Input: part model. Units: mm. Frame: model coordinates. A direction names the side the tool comes from. Coordinates: 2 decimals unless noted, no trailing zeros. Order: outer loops, then holes, each group sorted by start corner. A loop starts at its lowest first (then second) coordinate and runs counter-clockwise, first axis right, second up. Notation, with made-up numbers: (15.5, 12) -> (47.5, 12) arc R25 cw to (47.5, 37) -> close; hole circle Ø5 at (-25.5, 43). An arc over 180 degrees is marked (long way). One line per question, with ' | ' between items.
```python
from build123d import *

# Parameters (mm, degrees)
BOSS_EXTRUDE1_DEPTH = 100
SKETCH2_R           = 5
CUT_EXTRUDE1_DEPTH  = 61
BOSS_EXTRUDE3_DEPTH = 70
BOSS_EXTRUDE4_REACH = 124.997
SKETCH4_W           = 48
SKETCH4_H           = 70
CUT_EXTRUDE2_REACH  = 131.834
FILLET1_R           = 10
CUT_EXTRUDE3_DEPTH  = 56
FILLET3_R           = 18
FILLET4_R           = 15
FILLET5_R           = 15


with BuildPart() as part:
    # Sketch1 → Boss-Extrude1 (new body)
    with BuildSketch(Plane(origin=(0, 0, 0), x_dir=(0, 0, -1), z_dir=(1, 0, 0))):
        Polygon((9.31960102, -5.422823355), (-6.40194197, 19.363300607), (-0.164443236, 19.363300607), (44.235722397, -50.636699393), (37.998223663, -50.636699393), (29.951005386, -37.94969088), align=None)
    extrude(amount=BOSS_EXTRUDE1_DEPTH)

    # Sketch2 → Cut-Extrude1 (cut)
    with BuildSketch(Plane(origin=(0, 0, -44.235722397), x_dir=(-1, 0, 0), z_dir=(0, 0, -1))):
        with Locations(Location((-80, -41.23638567, 0), (0, 0, 270))):
            Circle(SKETCH2_R)
        with Locations(Location((-20, -41.23638567, 0), (0, 0, 270))):
            Circle(SKETCH2_R)
        with Locations(Location((-20, 8.76361433, 0), (0, 0, 270))):
            Circle(SKETCH2_R)
        with Locations(Location((-80, 8.76361433, 0), (0, 0, 270))):
            Circle(SKETCH2_R)
    extrude(amount=-CUT_EXTRUDE1_DEPTH, mode=Mode.SUBTRACT)

    # Boss-Extrude4: up to this face of the body (flat: up to its plane)
    boss_extrude4_end = Plane(part.part.faces().sort_by_distance((50, -15.608520887, -15.780267556))[0])
    # Sketch4 → Boss-Extrude4 (add, up to the picked face)
    with BuildSketch(Plane(origin=(0, 0, 6.40194197), x_dir=(-1, 0, 0), z_dir=(0, 0, -1)), mode=Mode.PRIVATE) as boss_extrude4_sk1:
        with Locations((-50, -15.636699393)):
            Rectangle(SKETCH4_W, SKETCH4_H)
    boss_extrude4_tool1 = split(extrude(boss_extrude4_sk1.sketch, amount=BOSS_EXTRUDE4_REACH, mode=Mode.PRIVATE), bisect_by=boss_extrude4_end, keep=Keep.BOTH, mode=Mode.PRIVATE)


with BuildPart() as body_2:
    # Sketch3 → Boss-Extrude3 (new body)
    with BuildSketch(Plane(origin=(0, 19.363300607, 0), x_dir=(1, 0, 0), z_dir=(0, 1, 0))):
        with BuildLine():
            Line((26, -6.40194197), (74, -6.40194197))
            ThreePointArc((74, -6.40194197), (50, -10.164443236), (26, -6.40194197))
        make_face()
    extrude(amount=-BOSS_EXTRUDE3_DEPTH)


with BuildPart() as part_1:
    add(part.part)

    add(body_2.part)  # Boss-Extrude4 merges body 2
    add(boss_extrude4_tool1.solids().sort_by(Axis((50, -15.636699, 6.401942), (0, 0, -1)))[0])

    # Cut-Extrude2: up to this face of the body (flat: up to its plane)
    cut_extrude2_end = Plane(part_1.part.faces().sort_by_distance((87.661220736, -15.580052964, -15.762210692))[0])
    # Sketch5 → Cut-Extrude2 (cut, up to the picked face)
    with BuildSketch(Plane.XZ.offset(50.636699393), mode=Mode.PRIVATE) as cut_extrude2_sk1:
        with BuildLine():
            Line((68.503998914, -37.998223663), (31.496001086, -37.998223663))
            Line((31.496001086, -37.998223663), (31.496001086, 4.779601344))
            ThreePointArc((31.496001086, 4.779601344), (50, 7.087022557), (68.503998914, 4.779601344))
            Line((68.503998914, 4.779601344), (68.503998914, -37.998223663))
        make_face()
    cut_extrude2_tool1 = split(extrude(cut_extrude2_sk1.sketch, amount=-CUT_EXTRUDE2_REACH, mode=Mode.PRIVATE), bisect_by=cut_extrude2_end, keep=Keep.BOTH, mode=Mode.PRIVATE)
    add(cut_extrude2_tool1.solids().sort_by(Axis((50, -50.636699, -15.832469), (0, 1, 0)))[0], mode=Mode.SUBTRACT)

    # Fillet1
    # the kernel refuses this fillet: 10 mm, written as the material it takes off along each edge
    with BuildSketch(Plane(origin=(100, -50.636699393, -69.235722397), x_dir=(-1, 0, 0), z_dir=(0, 0, 1)), Plane(origin=(100, 19.363300607, 31.40194197), x_dir=(-1, 0, 0), z_dir=(0, 0, -1))) as fillet1_piece_1:
        with BuildLine():
            CenterArc((FILLET1_R, -FILLET1_R), FILLET1_R, 90, 90)
            Line((0, -FILLET1_R), (0, 0))
            Line((0, 0), (FILLET1_R, 0))
        make_face()
    extrude(amount=56.237498734, mode=Mode.SUBTRACT)
    with BuildSketch(Plane(origin=(0, -50.636699393, -69.235722397), x_dir=(1, 0, 0), z_dir=(0, 0, 1)), Plane(origin=(0, 19.363300607, 31.40194197), x_dir=(1, 0, 0), z_dir=(0, 0, -1))) as fillet1_piece_2:
        with BuildLine():
            CenterArc((FILLET1_R, FILLET1_R), FILLET1_R, 180, 90)
            Line((0, FILLET1_R), (0, 0))
            Line((0, 0), (FILLET1_R, 0))
        make_face()
    extrude(amount=56.237498734, mode=Mode.SUBTRACT)

    # Sketch7 → Cut-Extrude3 (cut)
    with BuildSketch(Plane(origin=(74, 0, 0), x_dir=(0, 0, -1), z_dir=(1, 0, 0))):
        Polygon((5.879968804, 0), (-34.029101203, 0), (-34.029101203, -30), (24.908611218, -30), align=None)
    extrude(amount=-CUT_EXTRUDE3_DEPTH, mode=Mode.SUBTRACT)

    # Fillet3
    # the kernel refuses this fillet: 18 mm, written as the material it takes off along each edge
    with BuildSketch(Plane(origin=(74, 60.763896609, 6.40194197), x_dir=(-0.9790132085588953, 0, 0.20379680435967867), z_dir=(0, -1, 0))) as fillet3_piece_1_section:
        with BuildLine():
            CenterArc((14.659822692, 17.8993972), FILLET3_R, 191.759074187, 84.301431918)
            Line((-2.962415062, 14.231054722), (0, 0))
            ThreePointArc((0, 0), (8.2801192, -0.43832682), (16.560238401, 0))
        make_face()
    fillet3_piece_1 = extrude(amount=102.16449261, mode=Mode.PRIVATE)
    fillet3_piece_1 = split(fillet3_piece_1, bisect_by=Plane(origin=(69.993439145, 10.97404697, 1.080738384), z_dir=(0, -0.5356273864218708, 0.8444544409942292)), keep=Keep.TOP, mode=Mode.PRIVATE)
    add(fillet3_piece_1, mode=Mode.SUBTRACT)
    with BuildSketch(Plane(origin=(74, 11.400596002, 6.40194197), x_dir=(-0.9790132085588953, 0, 0.2037968043596786), z_dir=(0, -1, 0))) as fillet3_piece_2_section:
        with BuildLine():
            CenterArc((14.659822692, 17.8993972), FILLET3_R, 191.759074187, 84.301431918)
            Line((-2.962415062, 14.231054722), (0, 0))
            ThreePointArc((0, 0), (8.2801192, -0.43832682), (16.560238401, 0))
        make_face()
    fillet3_piece_2 = extrude(amount=103.437891396, mode=Mode.PRIVATE)
    fillet3_piece_2 = split(fillet3_piece_2, bisect_by=Plane(origin=(70.341248141, 8.727743457, -0.34406516), z_dir=(0, -0.5356273864218708, 0.8444544409942292)), keep=Keep.TOP, mode=Mode.PRIVATE)
    add(fillet3_piece_2, mode=Mode.SUBTRACT)
    with BuildSketch(Plane(origin=(26, 11.400596002, 6.40194197), x_dir=(0, 0, -1), z_dir=(0, -1, 0))) as fillet3_piece_3_section:
        with BuildLine():
            CenterArc((14.536121267, 18), FILLET3_R, 185.698568082, 84.301431918)
            ThreePointArc((-3.374923665, 16.212692131), (-2.116589579, 8.01701646), (0, 0))
            Line((0, 0), (14.536121267, 0))
        make_face()
    fillet3_piece_3 = extrude(amount=103.437891396, mode=Mode.PRIVATE)
    fillet3_piece_3 = split(fillet3_piece_3, bisect_by=Plane(origin=(29.658751859, 8.727743457, -0.344065159), z_dir=(0, -0.5356273864218708, 0.8444544409942292)), keep=Keep.TOP, mode=Mode.PRIVATE)
    add(fillet3_piece_3, mode=Mode.SUBTRACT)
    with BuildSketch(Plane(origin=(26, 60.763896609, 6.40194197), x_dir=(0, 0, -1), z_dir=(0, -1, 0))) as fillet3_piece_4_section:
        with BuildLine():
            CenterArc((14.536121267, 18), FILLET3_R, 185.698568082, 84.301431918)
            ThreePointArc((-3.374923665, 16.212692131), (-2.116589579, 8.01701646), (0, 0))
            Line((0, 0), (14.536121267, 0))
        make_face()
    fillet3_piece_4 = extrude(amount=102.16449261, mode=Mode.PRIVATE)
    fillet3_piece_4 = split(fillet3_piece_4, bisect_by=Plane(origin=(30.006560852, 10.974046968, 1.080738383), z_dir=(0, -0.5356273864218708, 0.8444544409942292)), keep=Keep.TOP, mode=Mode.PRIVATE)
    add(fillet3_piece_4, mode=Mode.SUBTRACT)

    # Fillet4
    fillet4_edges = [part_1.edges().sort_by_distance(p)[0] for p in [
        (68.503998914, -40.318349696, 4.779601344),
        (31.496001086, -40.318349696, 4.779601344),
    ]]
    fillet(fillet4_edges, radius=FILLET4_R)

    # Fillet5
    # the kernel refuses this fillet: 15 mm, written as the material it adds along each edge
    with BuildSketch(Plane(origin=(68.503998914, 0, 4.779601344), x_dir=(0, 0, -1), z_dir=(0, 1, 0))) as fillet5_piece_1_section:
        with BuildLine():
            CenterArc((12.794390285, 15), FILLET5_R, 183.32861315, 86.67138685)
            ThreePointArc((-2.18030389, 14.12906122), (-1.426006953, 7.012703672), (0, 0))
            Line((0, 0), (12.794390285, 0))
        make_face()
    fillet5_piece_1 = extrude(amount=52.546307376, mode=Mode.PRIVATE)
    fillet5_piece_1 = split(fillet5_piece_1, bisect_by=Plane(origin=(64.873583949, 12.366179926, -4.273747009), z_dir=(0, -0.5356273864218707, 0.8444544409942292)), keep=Keep.TOP, mode=Mode.PRIVATE)
    fillet5_piece_1 = split(fillet5_piece_1, bisect_by=Plane(origin=(64.873583949, 19.363300607, 3.531905566), z_dir=(0, -1, 0)), keep=Keep.TOP, mode=Mode.PRIVATE)
    add(fillet5_piece_1)
    with BuildSketch(Plane(origin=(31.496001086, 0, 4.779601344), x_dir=(0.9883021898179025, 0, 0.15250830010572736), z_dir=(0, 1, 0))) as fillet5_piece_2_section:
        with BuildLine():
            CenterArc((12.873282134, 14.932348438), FILLET5_R, 188.772314309, 86.67138685)
            Line((-1.951250713, 12.644723937), (0, 0))
            ThreePointArc((0, 0), (7.148148292, -0.339830278), (14.296296583, 0))
        make_face()
    fillet5_piece_2 = extrude(amount=52.546307376, mode=Mode.PRIVATE)
    fillet5_piece_2 = split(fillet5_piece_2, bisect_by=Plane(origin=(35.126416052, 12.366179929, -4.273747008), z_dir=(0, -0.5356273864218707, 0.8444544409942292)), keep=Keep.TOP, mode=Mode.PRIVATE)
    fillet5_piece_2 = split(fillet5_piece_2, bisect_by=Plane(origin=(35.126416052, 19.363300607, 3.531905566), z_dir=(0, -1, 0)), keep=Keep.TOP, mode=Mode.PRIVATE)
    add(fillet5_piece_2)


solid = part_1.part
```
1. Ray query, line 1 (X direction, y = -46.5, z = -28); line 2 (Z direction, x = 50.5, y = -38.5); line 3 (Z direction, x = 46, y = -33.5). Return the intervals inside material, ascending. Write a range as [from, to].
Recorded:
line 1: x = [26, 31.5], [68.5, 74] | line 2: z = [-36.54, -30.3], [7.09, 10.16] | line 3: z = [-33.37, -27.13], [6.98, 10.06]
2. Mould query, pull axis Z, two halves, no side actions, for faces 1 (the face through (68.504, -40, -19)), 2 (the face through (81.915, -45.855, -35.243)), 3 (the face through (50.109, 9.817, 10.164)). Classes: released by +Z, released by -Z, zero draft, split by the parting line, or undercut.
Recorded:
face 1: undercut | face 2: zero draft | face 3: released by +Z
3. Cut plane D-D, the plane x = 20. Return loops of the section in (y, z), and give its area (3 significant figures).
Recorded:
outline: (-50.64, -44.24) -> (-46.24, -41.44) -> (-46.24, -35.21) -> (-50.64, -38) -> close; (-36.24, -35.1) -> (3.76, -9.73) -> (3.76, -3.49) -> (-36.24, -28.86) -> close; (13.76, -3.39) -> (19.36, 0.16) -> (19.36, 6.4) -> (13.76, 2.85) -> close | area: 312 mm^2
4. Cut plane C-C, the plane z = -23.5. Return loops of the section in (x, y), and give its area (3 significant figures).
Recorded:
outline: (0, -27.78) -> (100, -27.78) -> (100, -17.95) -> (0, -17.95) -> close; (26, -50.64) -> (31.5, -50.64) -> (31.5, -30) -> (26, -30) -> close; (68.5, -50.64) -> (74, -50.64) -> (74, -30) -> (68.5, -30) -> close | area: 1,210 mm^2
5. Pin query (flat end, axial travel): pin 1 Ø8 at (x, y) = (80, 8.76) entering from -Z; pin 2 Ø4 at (x, z) = (17, -28) entering from -Y; pin 3 Ø12 at (x, z) = (70.5, -8.5) entering from +Y; pin 4 Ø8 at (x, y) = (62.5, -12.5) entering from -Z. Return the tip coordinate at first contact, or that it passes through.
Recorded:
pin 1: passes through | pin 2: stops at y = -37.84 | pin 3: stops at y = 15.16 | pin 4: stops at z = -22.58
6. Cut plane B-B, the plane y = 1.5. Return loops of the section in (x, z), and give its area (3 significant figures).
Recorded:
outline: (0, -11.17) -> (100, -11.17) -> (100, -4.93) -> (73.71, -4.93) arc R18 ccw to (57.79, 9.78) arc R78.43 ccw to (42.21, 9.78) arc R18 ccw to (26.29, -4.93) -> (0, -4.93) -> close; hole (31.82, -4.93) -> (68.18, -4.93) arc R15 ccw to (54.37, 6.96) arc R75.35 ccw to (45.63, 6.96) arc R15 ccw to start | area: 853 mm^2
7. Access query for faces 4 (the face through (48.1, 0, 7.5)), 5 (the face through (49.939, -40.463, 7.087)), 6 (the face through (30.78, -40.17, 4.08)), 7 (the face through (64.3, -40.2, 2.4)). Directions: +Z, -Z, +X, -X, +Y, -Y. A direction counts if a zero-diameter tool reaches every point of the face in a straight line with its end or side. Return the directions, or none.
Recorded:
face 4: +Z, +X, -X | face 5: +Y, -Y | face 6: +Z, -X, -Y | face 7: -Y
8. Cut plane A-A, the plane x = 40. Return loops of the section in (y, z).
Recorded:
outline: (-50.64, -44.24) -> (19.36, 0.16) -> (19.36, 9.42) -> (0, 9.42) -> (0, 5.51) -> (17.95, 5.51) -> (-50.64, -38) -> close; (-50.64, 5.51) -> (-30, 5.51) -> (-30, 9.42) -> (-50.64, 9.42) -> close
